from build123d import *
from build123d import SkipClean  # not in build123d's __all__

# Parameters (mm, degrees)
F0_W      = 20
F0_H      = 90
F1_DEPTH  = 18
F4_W      = 11.5
F4_H      = 4.5
F4_H_2    = 2
F6_REACH  = 51.4753785472
F8_W      = 43.5633249581
F8_H      = 43.13050583
F9_DEPTH  = 16.4
F10_R     = 3
F12_DEPTH = 7
F13_DEPTH = 1


with BuildPart() as f1:
    # F0 (on Front) → F1 (new body)
    with BuildSketch(Plane.XZ):
        Rectangle(F0_W, F0_H)
    extrude(amount=F1_DEPTH)

    f6_end = Plane(origin=(0, -8, 0), x_dir=(0, 0, -1), z_dir=(0, -1, 0))
    # F4 (on face) → F6 (cut, up to a plane its end follows)
    with BuildSketch(Plane(origin=(0, -30.357121206, 11.049088517), x_dir=(-1, 0, 0), z_dir=(0, 0.9396926208, -0.3420201433))):
        with Locations((0, 24.6185707509)):
            Rectangle(F4_W, F4_H)
        with Locations((0, 10.1185707509)):
            Rectangle(F4_W, F4_H)
        with Locations((0, -4.3814292491)):
            Rectangle(F4_W, F4_H)
        with Locations((0, -18.8814292491)):
            Rectangle(F4_W, F4_H)
        with Locations((0, -26.1314292491)):
            Rectangle(F4_W, F4_H_2)
        with Locations((0.0476672364, -31.1312020274)):
            Rectangle(F4_W, F4_H_2)
        with Locations((0.0953344728, -36.1309748057)):
            Rectangle(F4_W, F4_H_2)
        with Locations((0.1430017093, -41.130747584)):
            Rectangle(F4_W, F4_H_2)
    f6_long = extrude(amount=F6_REACH, mode=Mode.PRIVATE)
    add(split(f6_long, bisect_by=f6_end, keep=Keep.TOP, mode=Mode.PRIVATE), mode=Mode.SUBTRACT)

    # F8 (on offset) → F9 (cut)
    with BuildSketch(Plane(origin=(0, 12.2677737091, 33.7054312527), x_dir=(1, 0, 0), z_dir=(0, -0.3420201433, -0.9396926208))):
        with Locations((0, 21.565252915)):
            Rectangle(F8_W, F8_H)
    extrude(amount=-F9_DEPTH, mode=Mode.SUBTRACT)

    # F10
    f10_edges = [f1.edges().sort_by_distance(p)[0] for p in [
        (-10, -18, -0.139),
        (0, -18, 44.722),
        (10, -18, -0.139),
        (0, -18, -45),
        (-10, -9, 41.446268),
        (10, -9, 41.446268),
        (-10, -9, -45),
        (10, -9, -45),
    ]]
    fillet(f10_edges, radius=F10_R)

    # F11 (on face) → F12 (cut)
    with BuildSketch(Plane(origin=(0, 0, 0), x_dir=(-1, 0, 0), z_dir=(0, 1, 0))):
        with BuildLine():
            ThreePointArc((-5.25, 20), (0, 14.75), (5.25, 20))
            ThreePointArc((5.25, 20), (4.9157552788, 21.8433258091), (3.9555809377, 23.4519385054))
            ThreePointArc((3.9555809377, 23.4519385054), (0, 25.25), (-3.9555809377, 23.4519385054))
            ThreePointArc((-3.9555809377, 23.4519385054), (-4.9157552788, 21.8433258091), (-5.25, 20))
        make_face()
        with BuildLine():
            ThreePointArc((3.9555809377, 23.4519385054), (4.9157552788, 21.8433258091), (5.25, 20))
            Line((5.25, 20), (5.25, 32.8980128765))
            ThreePointArc((5.25, 32.8980128765), (4.6642135624, 34.3122264389), (3.25, 34.8980128765))
            Line((3.25, 34.8980128765), (-3.25, 34.8980128765))
            ThreePointArc((-3.25, 34.8980128765), (-4.6642135624, 34.3122264389), (-5.25, 32.8980128765))
            Line((-5.25, 32.8980128765), (-5.25, 20))
            ThreePointArc((-5.25, 20), (-4.9157552788, 21.8433258091), (-3.9555809377, 23.4519385054))
            Line((-3.9555809377, 23.4519385054), (-3.9555809377, 31.6754657328))
            ThreePointArc((-3.9555809377, 31.6754657328), (-3.3697945001, 33.0896792952), (-1.9555809377, 33.6754657328))
            Line((-1.9555809377, 33.6754657328), (1.9555809377, 33.6754657328))
            ThreePointArc((1.9555809377, 33.6754657328), (3.3697945001, 33.0896792952), (3.9555809377, 31.6754657328))
            Line((3.9555809377, 31.6754657328), (3.9555809377, 23.4519385054))
        make_face()
        with BuildLine():
            ThreePointArc((-3.9555809377, 23.4519385054), (0, 25.25), (3.9555809377, 23.4519385054))
            Line((3.9555809377, 23.4519385054), (3.9555809377, 31.6754657328))
            ThreePointArc((3.9555809377, 31.6754657328), (3.3697945001, 33.0896792952), (1.9555809377, 33.6754657328))
            Line((1.9555809377, 33.6754657328), (-1.9555809377, 33.6754657328))
            ThreePointArc((-1.9555809377, 33.6754657328), (-3.3697945001, 33.0896792952), (-3.9555809377, 31.6754657328))
            Line((-3.9555809377, 31.6754657328), (-3.9555809377, 23.4519385054))
        make_face()
    extrude(amount=-F12_DEPTH, mode=Mode.SUBTRACT)

    # F11 (on face) → F13 (join)
    with BuildSketch(Plane(origin=(0, 0, 0), x_dir=(-1, 0, 0), z_dir=(0, 1, 0))):
        with BuildLine():
            ThreePointArc((3.9555809377, 23.4519385054), (4.9157552788, 21.8433258091), (5.25, 20))
            Line((5.25, 20), (5.25, 32.8980128765))
            ThreePointArc((5.25, 32.8980128765), (4.6642135624, 34.3122264389), (3.25, 34.8980128765))
            Line((3.25, 34.8980128765), (-3.25, 34.8980128765))
            ThreePointArc((-3.25, 34.8980128765), (-4.6642135624, 34.3122264389), (-5.25, 32.8980128765))
            Line((-5.25, 32.8980128765), (-5.25, 20))
            ThreePointArc((-5.25, 20), (-4.9157552788, 21.8433258091), (-3.9555809377, 23.4519385054))
            Line((-3.9555809377, 23.4519385054), (-3.9555809377, 31.6754657328))
            ThreePointArc((-3.9555809377, 31.6754657328), (-3.3697945001, 33.0896792952), (-1.9555809377, 33.6754657328))
            Line((-1.9555809377, 33.6754657328), (1.9555809377, 33.6754657328))
            ThreePointArc((1.9555809377, 33.6754657328), (3.3697945001, 33.0896792952), (3.9555809377, 31.6754657328))
            Line((3.9555809377, 31.6754657328), (3.9555809377, 23.4519385054))
        make_face()
    with SkipClean():  # cleaning this boolean's faces spoils the solid; the shape is the same uncleaned
        extrude(amount=-F13_DEPTH)


solid = f1.part
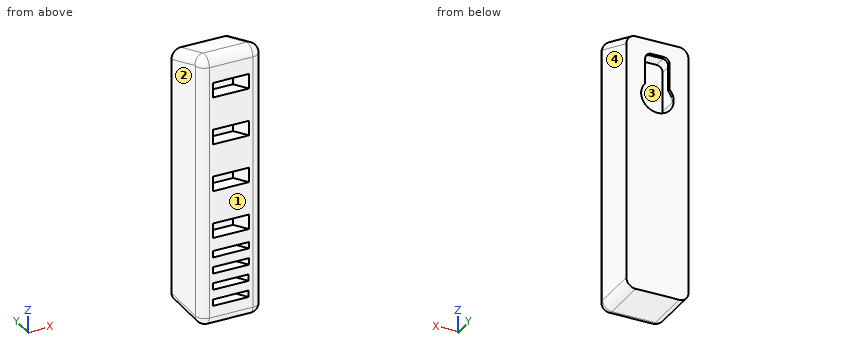
For this review, take the finished solid that the model builds, in its own axes (mm). Face numbers are marked on the shaded views. Round coordinates to 2 decimals unless told otherwise and drop trailing zeros. Use a Markdown table: item, result. Add a question column.
Item 1: Insertion check: pin 1 (1 mm diameter, centred on x = -8, z = 33, fed in from -Y); pin 2 (3 mm diameter, centred on x = -1.5, y = -3.5, fed in from +Z). Each pin has a flat end and moves straight along its axis. Give the tip position at first contact, or say it passes through.
Item 2: Mouldability with a two-part tool opening along X and no side actions: class the marked faces 1, 2, 3 and 4 as released by +X, released by -X, zero draft, split by the parting line, or undercut.
Item 3: To check wall thickness, follow line 1 along X through (y, z) = (-12.5, -1); line 2 along Y through (x, z) = (7.25, 30); line 3 along X through (y, z) = (-16, 31). State the ranges of each line that lie inside material, in increasing order.
Geometry results:
| question | item | result |
|---|---|---|
| 1 | pin 1 | stops at y = -17.96 |
| 1 | pin 2 | stops at z = 39.99 |
| 2 | face 1 | zero draft |
| 2 | face 2 | released by -X |
| 2 | face 3 | undercut |
| 2 | face 4 | released by +X |
| 3 | line 1 | x = -10 to -5.75, 5.75 to 10 |
| 3 | line 2 | y = -17.99 to 0 |
| 3 | line 3 | x = -9.83 to -5.75, 5.75 to 9.83 |
